from build123d import *

# Parameters (mm, degrees)
SKETCH1_W           = 12
SKETCH1_H           = 12
SKETCH1_R           = 2.75
BOSS_EXTRUDE1_DEPTH = 4
SKETCH2_W           = 4
SKETCH2_H           = 10
BOSS_EXTRUDE2_DEPTH = 22
SKETCH3_W           = 4
SKETCH3_H           = 12
BOSS_EXTRUDE3_DEPTH = 10
SKETCH4_R           = 1.1
CUT_EXTRUDE1_DEPTH  = 18
FILLET1_R           = 5.5
FILLET2_R           = 3


with BuildPart() as part:
    # Sketch1 → Boss-Extrude1 (new body)
    # profile 1 of 4: a face of its own
    with BuildSketch(Plane.XY):
        Polygon((9, 6), (9, 0), (9, -6), (21, -6), (21, 6), align=None)
        with BuildLine():
            ThreePointArc((17.75, 0), (15, -2.75), (12.25, 0))
            ThreePointArc((12.25, 0), (15, 2.75), (17.75, 0))
        make_face(mode=Mode.SUBTRACT)
    # profile 2 of 4: a face of its own
    with BuildSketch(Plane.XY):
        Polygon((0, 6), (9, 6), (21, 6), (21, 16), (0, 16), align=None)
    # profile 3 of 4: a face of its own
    with BuildSketch(Plane.XY):
        Polygon((-9, 6), (0, 6), (0, 16), (-21, 16), (-21, 6), align=None)
    # profile 4 of 4: a face of its own
    with BuildSketch(Plane.XY):
        with Locations((-15, 0)):
            Rectangle(SKETCH1_W, SKETCH1_H)
        with Locations((-15, 0)):
            Circle(SKETCH1_R, mode=Mode.SUBTRACT)
    extrude(amount=BOSS_EXTRUDE1_DEPTH)

    # Sketch2 → Boss-Extrude2 (add)
    with BuildSketch(Plane.XY.offset(4)):
        with Locations((4, 11)):
            Rectangle(SKETCH2_W, SKETCH2_H)
    extrude(amount=BOSS_EXTRUDE2_DEPTH)

    # Sketch3 → Boss-Extrude3 (add)
    with BuildSketch(Plane.XZ.offset(-6)):
        with Locations((4, 20)):
            Rectangle(SKETCH3_W, SKETCH3_H)
    extrude(amount=BOSS_EXTRUDE3_DEPTH)

    # Sketch4 → Cut-Extrude1 (cut)
    with BuildSketch(Plane.ZY.offset(-2)):
        with Locations((23.25, -1)):
            Circle(SKETCH4_R)
        with Locations((16.75, -1)):
            Circle(SKETCH4_R)
    extrude(amount=-CUT_EXTRUDE1_DEPTH, mode=Mode.SUBTRACT)

    # Fillet1
    fillet1_edges = [part.edges().sort_by_distance(p)[0] for p in [
        (-21, 16, 2),
        (21, 16, 2),
        (21, -6, 2),
        (9, -6, 2),
        (9, 6, 2),
        (-9, 6, 2),
        (-9, -6, 2),
        (-21, -6, 2),
    ]]
    fillet(fillet1_edges, radius=FILLET1_R)

    # Fillet2
    fillet2_edges = [part.edges().sort_by_distance(p)[0] for p in [
        (2.75, 6, 14),
        (4.785615189, 5.847634392, 14),
        (6, 10.699489743, 4),
        (2, 11, 4),
        (4, 16, 26),
        (4, -4, 26),
        (4, -4, 14),
    ]]
    fillet(fillet2_edges, radius=FILLET2_R - 0.0001)  # a hair under: the kernel refuses the full size


solid = part.part
Check sheet for the modelled part. Datum: model origin and axes. Units: mm. A direction names the side the tool comes from. Round coordinates to 2 decimals unless told otherwise and drop trailing zeros. Write each loop counter-clockwise with the first axis right and the second up, starting at its lowest first coordinate (ties: lowest second). Pieces come first, ordered by that corner, then holes. Notation, with made-up numbers: (3.5, 44.5) - (19.5, 44.5) arc R20 cw to (19.5, 54.5) - close; hole circle Ø5 at (52.25, 31.25). An arc over 180 degrees is marked (long way). Return JSON: item names as keys, results as strings.
Q1. Cross-section at B-B (z = 2.5). Record the boundary of the cut face in (x, y).
Returned:
{"outline": "(-21, -0.5) arc R5.5 ccw to (-15.5, -6) - (-14.5, -6) arc R5.5 ccw to (-9, -0.5) - (-9, 0.5) arc R5.5 cw to (-3.5, 6) - (3.5, 6) arc R5.5 cw to (9, 0.5) - (9, -0.5) arc R5.5 ccw to (14.5, -6) - (15.5, -6) arc R5.5 ccw to (21, -0.5) - (21, 10.5) arc R5.5 ccw to (15.5, 16) - (-15.5, 16) arc R5.5 ccw to (-21, 10.5) - close; hole circle Ø5.5 at (-15, 0); hole circle Ø5.5 at (15, 0)"}
Q2. Access from +Z, -Z, +X, -X, +Y, -Y to the whole of each face (thin tool, end or side, straight path). Record for faces 1 (the flat face through (-13, 8, 4)), 2 (the flat face through (6, 8, 18)), 3 (the flat face through (4, 1, 14)).
Returned:
{"face 1": "+Z, -X, +Y, -Y", "face 2": "+Z, +X, +Y, -Y", "face 3": "-Z, -X, -Y"}
Q3. Cross-section at C-C (y = 8.5). Record the boundary of the cut face in (x, z).
Returned:
{"outline": "(-21, 0) - (21, 0) - (21, 4) - (9, 4) arc R3 cw to (6, 7) - (6, 26) - (2, 26) - (2, 7) arc R3 cw to (-1, 4) - (-21, 4) - close"}
Q4. Cross-section at A-A (x = -15). Record the boundary of the cut face in (y, z).
Returned:
{"outline": "(-6, 0) - (-2.75, 0) - (-2.75, 4) - (-6, 4) - close; (2.75, 0) - (16, 0) - (16, 4) - (2.75, 4) - close"}
Q5. Depth check by flat-ended pin: P1, Ø6.5, axis at x = -15, y = 0, coming from the +Z side; P2, Ø4, axis at y = 4, z = 14.5, coming from the +X side; P3, Ø3, axis at x = 4.5, z = 20, coming from the -Y side. Enter the tip coordinate at first touch or a pass-through.
Returned:
{"P1": "stops at z = 4", "P2": "stops at x = 6", "P3": "stops at y = -4"}
Q6. Draft check along Y on faces 4 (the flat face through (9, 0, 2)), 5 (the cylindrical face through (3.97, -0.95, 22.15)), 6 (the cylindrical face through (17.747, 0.121, 1.972)), 7 (the cylindrical face through (6.605, 5.04, 4.355)). Enter one of: released by +Y, released by -Y, zero draft, split by the parting line, or undercut.
Returned:
{"face 4": "zero draft", "face 5": "undercut", "face 6": "undercut", "face 7": "released by -Y"}
Q7. Cross-section at D-D (z = 16.5). Record the boundary of the cut face in (x, y).
Returned:
{"outline": "(2, -3.96) - (6, -3.96) - (6, -2.07) - (2, -2.07) - close; (2, 0.07) - (6, 0.07) - (6, 16) - (2, 16) - close"}
Q8. Scan lines: L1, parallel to Y at x = 15, z = 1.4; L2, parallel to Y at x = 4.8, z = 16.75; L3, parallel to X at y = 5.75, z = 13.75. Record each from-to range of solid material in increasing order. Write a range as from..to.
Returned:
{"L1": "y = -6..-2.75, 2.75..16", "L2": "y = -3.99..-2.1, 0.1..16", "L3": "x = 2..6"}
